```python
from build123d import *

# Parameters (mm, degrees)
F0_R     = 5
F1_DEPTH = 12


with BuildPart() as f1:
    # F0 (on Front) → F1 (new body)
    with BuildSketch(Plane.XZ):
        with BuildLine():
            Line((44.5, 33.5), (-44.5, 33.5))
            ThreePointArc((-44.5, 33.5), (-51.571068, 30.571068), (-54.5, 23.5))
            Line((-54.5, 23.5), (-54.5, -23.5))
            ThreePointArc((-54.5, -23.5), (-51.571068, -30.571068), (-44.5, -33.5))
            Line((-44.5, -33.5), (44.5, -33.5))
            ThreePointArc((44.5, -33.5), (51.571068, -30.571068), (54.5, -23.5))
            Line((54.5, -23.5), (54.5, 23.5))
            ThreePointArc((54.5, 23.5), (51.571068, 30.571068), (44.5, 33.5))
        make_face()
        with Locations((-44.5, -23.5)):
            Circle(F0_R, mode=Mode.SUBTRACT)
        with Locations((44.5, -23.5)):
            Circle(F0_R, mode=Mode.SUBTRACT)
        with BuildLine():
            Line((-2.5, 13), (-2.5, 0))
            Line((-2.5, 0), (-2.5, -13))
            ThreePointArc((-2.5, -13), (-5.428932, -20.071068), (-12.5, -23))
            Line((-12.5, -23), (-22.5, -23))
            ThreePointArc((-22.5, -23), (-29.571068, -20.071068), (-32.5, -13))
            Line((-32.5, -13), (-32.5, 0))
            Line((-32.5, 0), (-32.5, 13))
            ThreePointArc((-32.5, 13), (-29.571068, 20.071068), (-22.5, 23))
            Line((-22.5, 23), (-12.5, 23))
            ThreePointArc((-12.5, 23), (-5.428932, 20.071068), (-2.5, 13))
        make_face(mode=Mode.SUBTRACT)
        with Locations((-44.5, 23.5)):
            Circle(F0_R, mode=Mode.SUBTRACT)
        with BuildLine():
            ThreePointArc((22.5, 23), (29.571068, 20.071068), (32.5, 13))
            Line((32.5, 13), (32.5, -13))
            ThreePointArc((32.5, -13), (29.571068, -20.071068), (22.5, -23))
            Line((22.5, -23), (12.5, -23))
            ThreePointArc((12.5, -23), (5.428932, -20.071068), (2.5, -13))
            Line((2.5, -13), (2.5, 0))
            Line((2.5, 0), (2.5, 13))
            ThreePointArc((2.5, 13), (5.428932, 20.071068), (12.5, 23))
            Line((12.5, 23), (22.5, 23))
        make_face(mode=Mode.SUBTRACT)
        with Locations((44.5, 23.5)):
            Circle(F0_R, mode=Mode.SUBTRACT)
    extrude(amount=F1_DEPTH)


solid = f1.part
```
Geometry check sheet. Reference: the model listing, model coordinates, mm. A direction names the side the tool comes from. Coordinates: 2 decimals unless noted, no trailing zeros. Loops run counter-clockwise (first coordinate to the right, second up) from the corner with the lowest first, then second, coordinate; pieces in that order, holes last.
Item 1: Sectioned sample at D-D, the plane x = -47. Record the boundary of the cut face in (y, z), then the cut area to 3 significant figures.
Item 2: Thickness scan on line 1 (X direction, y = -2, z = 11); line 2 (Z direction, x = -44.5, y = -4.25); line 3 (X direction, y = -6.75, z = -16). Record the ranges inside material, lowest first.
Item 3: Access from +Z, -Z, +X, -X, +Y, -Y to the whole of each face (thin tool, end or side, straight path). Record for faces 5 (the face through (-51.49, -5.92, 30.65)), 6 (the face through (-32.5, -6, 0)).
Item 4: Sectioned sample at B-B, the plane y = -10.25. Record the boundary of the cut face in (x, z), then the cut area to 3 significant figures.
Item 5: Sectioned sample at A-A, the plane z = 5. Record the boundary of the cut face in (x, y).
Item 6: Sectioned sample at C-C, the plane x = 30.5. Record the boundary of the cut face in (y, z).
Item 7: Go/stop test with a flat-tipped pin: pin 1 Ø8 at (x, z) = (-44.5, 23.5) entering from -Y. Record where the tip stops, or that it passes through.
Item 8: Release check for a two-part mould opening along Z. For faces 1 (the face through (1, -6, 33.5)), 2 (the face through (51.49, -5.92, -30.65)), 3 (the face through (-1, -12, 0)), 4 (the face through (-2.5, -6, 0)) record: released by +Z, released by -Z, zero draft, split by the parting line, or undercut.
Check result:
1. outline: (-12, -33.18) - (0, -33.18) - (0, -27.83) - (-12, -27.83) - close; (-12, -19.17) - (0, -19.17) - (0, 19.17) - (-12, 19.17) - close; (-12, 27.83) - (0, 27.83) - (0, 33.18) - (-12, 33.18) - close
1. area: 589 mm2
2. line 1: x = -54.5 to -32.5, -2.5 to 2.5, 32.5 to 54.5
2. line 2: z = -33.5 to -28.5, -18.5 to 18.5, 28.5 to 33.5
2. line 3: x = -54.5 to -32.04, -2.96 to 2.96, 32.04 to 54.5
3. face 5: +Z, -X, +Y, -Y
3. face 6: +Y, -Y
4. outline: (-54.5, -23.5) arc R10 ccw to (-44.5, -33.5) - (44.5, -33.5) arc R10 ccw to (54.5, -23.5) - (54.5, 23.5) arc R10 ccw to (44.5, 33.5) - (-44.5, 33.5) arc R10 ccw to (-54.5, 23.5) - close; hole circle Ø10 at (-44.5, -23.5); hole circle Ø10 at (-44.5, 23.5); hole (-32.5, -13) arc R10 ccw to (-22.5, -23) - (-12.5, -23) arc R10 ccw to (-2.5, -13) - (-2.5, 13) arc R10 ccw to (-12.5, 23) - (-22.5, 23) arc R10 ccw to (-32.5, 13) - close; hole (2.5, -13) arc R10 ccw to (12.5, -23) - (22.5, -23) arc R10 ccw to (32.5, -13) - (32.5, 13) arc R10 ccw to (22.5, 23) - (12.5, 23) arc R10 ccw to (2.5, 13) - close; hole circle Ø10 at (44.5, -23.5); hole circle Ø10 at (44.5, 23.5)
4. area: 4,310 mm2
5. outline: (-54.5, -12) - (-32.5, -12) - (-32.5, 0) - (-54.5, 0) - close; (-2.5, -12) - (2.5, -12) - (2.5, 0) - (-2.5, 0) - close; (32.5, -12) - (54.5, -12) - (54.5, 0) - (32.5, 0) - close
6. outline: (-12, -33.5) - (0, -33.5) - (0, -19) - (-12, -19) - close; (-12, 19) - (0, 19) - (0, 33.5) - (-12, 33.5) - close
7. pin 1: passes through
8. face 1: released by +Z
8. face 2: released by -Z
8. face 3: zero draft
8. face 4: undercut
